Input: part model. Units: mm. Frame: model coordinates. A direction names the side the tool comes from. Coordinates: 2 decimals unless noted, no trailing zeros. Loops run counter-clockwise (first coordinate to the right, second up) from the corner with the lowest first, then second, coordinate; pieces in that order, holes last.
(1) Mould query, pull axis X, two halves, no side actions, for faces 1 (the face through (-18.516, -32.709, 1.61)), 2 (the face through (-38.944, 18.34, 1.61)), 3 (the face through (-0.72, -32.66, 1.61)). Classes: released by +X, released by -X, zero draft, split by the parting line, or undercut.
(2) Contact query for flat-ended pins moving along their axis: P1, Ø1.7, axis at x = -2.38, y = 19.05, coming from the +Z side; P2, Ø1.6, axis at x = -11, z = 1.5, coming from the +Y side; P3, Ø1, axis at y = 69.5, z = 1.5, coming from the -X side; P4, Ø1.5, axis at x = -13, z = 0.5, coming from the +Y side. Output: stop coordinate, or through.
(3) Line query: L1, parallel to Y at x = -24.5, z = 0.35; L2, parallel to Y at x = -29, z = 1.6; L3, parallel to X at y = 77.5, z = 1.8. Output: solid intervals per line, ascending.
(4) Section B-B, the plane y = 69.85. Return loops of the section in (x, z) (1 decimal), then the cut area to 3 significant figures.
(5) Section A-A, the plane y = -16. Return loops of the section in (x, z) (1 decimal), then the cut area to 3 significant figures.
(6) Section C-C, the plane z = 2.4. Give the number of separate pieces and of enclosed holes in the cut face, then the cut area to 3 significant figures.
(7) Set-up query: faces 4 (the face through (-10, -29.206, 2)), 5 (the face through (-21.964, 82.011, 1.565)). Return all of +Z, -Z, +X, -X, +Y, -Y with unobstructed straight access to the full face (end or side cutting, diameter ignored); none if empty.
Autodesk Inventor part; units mm, degrees
ref_plane "YZ Plane" through (0, 0, 0) normal (1, 0, 0) x (0, 1, 0)
ref_plane "XZ Plane" through (0, 0, 0) normal (0, 1, 0) x (-1, 0, 0)
ref_plane "XY Plane" through (0, 0, 0) normal (0, 0, 1) x (1, 0, 0)
sketch "Sketch1" plane through (0, 0, 0) normal (0, 0, 1) x (1, 0, 0)
  line L0 (0, 0) -> (0, 136.2362)
  line L1 (-14.9636, 12.2907) -> (-39.7615, 17.7883)
  line L2 (-39.7615, 17.7883) -> (-33.7485, 44.911)
  line L3 (-33.7485, 44.911) -> (-8.9506, 39.4135)
  line L4 (-8.9506, 39.4135) -> (-14.9636, 12.2907)
  line L5 (-39.7615, 17.7883) -> (-8.9506, 39.4135) construction
  line L6 (-33.7485, 44.911) -> (-14.9636, 12.2907) construction
  circle A0 centre (-57.15, 12.7) radius 3.3401
  circle A1 centre (-57.15, 12.7) radius 6.35
  line L7 (0, 0) -> (-57.847, 6.3884)
  line L8 (-62.7825, 15.6321) -> (0, 136.2362)
  line L9 (-21.3496, 42.1622) -> (-27.3626, 15.0395) construction
  line L10 (0, 104.775) -> (-14.6831, 108.0302)
  line L11 (-35.4518, 7.8896) -> (-23.0529, 5.1408)
  line L12 (-23.0529, 5.1408) -> (-24.4273, -1.0586) construction
  line L13 (-24.4273, -1.0586) -> (-36.8262, 1.6901) construction
  line L14 (-36.8262, 1.6901) -> (-35.4518, 7.8896) construction
  line L15 (-35.4518, 7.8896) -> (-40.7688, 4.5023)
  line L16 (-8.9506, 39.4135) -> (-33.7485, 44.911)
  line L17 (-56.4271, 15.9609) -> (-57.15, 12.7) construction
  line L18 (-57.15, 12.7) -> (-60.4109, 13.4229) construction
  line L19 (-29.2523, 6.5152) -> (-36.1243, -24.4822) construction
  line L20 (-56.356, 15.9443) -> (-9.0672, 106.7852)
  line L21 (-35.1857, 56.612) -> (0, 48.8115)
  line L22 (-4.7625, 49.8673) -> (-4.7625, 105.8308)
  line L23 (-30.3721, 55.5448) -> (-10.3247, 94.0556)
  line L24 (-10.3247, 94.0556) -> (-4.7625, 92.8225)
  circle A2 centre (-17.3978, 7.9523) radius 2
  line L25 (0, 13.4938) -> (-4.7625, 13.4937) construction
  line L26 (-4.7625, 13.4937) -> (-4.7625, 24.6063) construction
  line L27 (-4.7625, 24.6063) -> (0, 24.6063) construction
  line L28 (0, 24.6063) -> (0, 13.4938) construction
  line L29 (-4.7625, 19.05) -> (0, 19.05) construction
  circle A3 centre (-2.3812, 19.05) radius 1.4224
  line L30 (-4.7625, 57.15) -> (0, 57.15) construction
  circle A4 centre (-2.3813, 57.15) radius 1.4224
  circle A5 centre (-2.3813, 63.5) radius 1.4224
  circle A6 centre (-2.3813, 69.85) radius 1.4224
  circle A7 centre (-2.3813, 76.2) radius 1.4224
  line L31 (-22.792, 92.4532) -> (-17.8635, 89.8876)
  circle A8 centre (-57.15, 12.7) radius 9.525 construction
  line L32 (-14.7625, 0.7937) -> (-4.7625, 0.7938)
  line L33 (-4.7625, 0.7938) -> (-4.7625, -29.2062)
  line L34 (-4.7625, -29.2062) -> (-14.7625, -29.2062)
  line L35 (-14.7625, -29.2062) -> (-14.7625, 0.7937)
  line L36 (-14.7625, 0.7937) -> (-4.7625, -29.2062) construction
  line L37 (-4.7625, 0.7938) -> (-14.7625, -29.2062) construction
  line L38 (-19.05, -33.3375) -> (0, -33.3375)
  line L39 (0, -33.3375) -> (0, 0)
  line L40 (-23.0529, 5.1408) -> (-19.05, -33.3375)
  circle A9 centre (-17.3978, 7.9523) radius 6.5 construction
  line L41 (-22.7129, 14.0087) -> (-24.6027, 5.4844) construction
  line L42 (-17.3978, 7.9523) -> (-23.8273, 9.3776) construction
  line L43 (-33.8287, 59.2189) -> (-45.835, 5.0618)
  point P0 (-24.3561, 28.6009)
  point P1 (-23.6144, 2.6079)
  point P2 (-36.3119, 4.0101)
  point P3 (-54.945, 18.6549)
  point P4 (0, 48.8115)
  point P5 (-24.3561, 28.6009)
  point P6 (-9.7625, -14.2062)
  dimension "d14" = 27.7812
  dimension "d15" = 25.4
  dimension "d16" = 12.5
  dimension "d17" = 6.6802
  dimension "d19" = 57.15
  dimension "d22" = 12.7
  dimension "d26" = 102.5
  dimension "d29" = 6.35
  dimension "d31" = 6.35
  dimension "d35" = 28.575
  dimension "d38" = 31.75
  dimension "d55" = 4.7625
  dimension "d56" = 4.7625
  dimension "d60" = 12.7
  dimension "d66" = 4
  dimension "d72" = 8.7312
  dimension "d80" = 104.775
  dimension "d85" = 4.7625
  dimension "d86" = 11.1125
  dimension "d87" = 2.8448
  dimension "d88" = 19.05
  dimension "d89" = 2.8448
  dimension "d90" = 38.1
  dimension "d93" = 6.35
  dimension "d104" = 27.5
  dimension "d105" = 5.5563
  dimension "d106" = 19.05
  dimension "d111" = 19.05
  dimension "d112" = 10
  dimension "d113" = 30
  dimension "d114" = 4.7625
  dimension "d115" = 0.7937
  dimension "d117" = 19.05
  dimension "d119" = 11.1125
  dimension "d120" = 12.7
  dimension "d121" = 33.3375
  dimension "d122" = 45
  dimension "d123" = 13
  dimension "d124" = 4.7625
  dimension "d125" = 4.7625
  dimension "d126" = 3.175
extrude "Extrusion1" add sketch "Sketch1" along normal blind 3.175 contours L7 L33 L32 L40 L11 L15 L43 L21 L0 | L39 L38 L40 L7 L32 L35 L34 L33 | L21 L22 L10 L0 | L22 L24 L23 L21 L43 L20 L10
fillet "Fillet1" radius 2.3813 17 edges at (-39.7615, 17.7883, 1.5875) (-14.9636, 12.2907, 1.5875) (-23.0529, 5.1408, 1.5875) (-35.4518, 7.8896, 1.5875) (-40.7688, 4.5023, 1.5875) (-4.7625, 92.8225, 1.5875) (-30.3721, 55.5448, 1.5875) (-4.7625, 49.8673, 1.5875) (-33.7485, 44.911, 1.5875) (-8.9506, 39.4135, 1.5875) (-19.05, -33.3375, 1.5875) (0, -33.3375, 1.5875) (-10.3247, 94.0556, 1.5875) (-33.8287, 59.2189, 1.5875) (-45.835, 5.0618, 1.5875) (-9.0672, 106.7852, 1.5875) (0, 104.775, 1.5875)
fillet "Fillet6" radius 1 4 edges at (-4.7625, 0.7938, 1.5875) (-14.7625, 0.7937, 1.5875) (-14.7625, -29.2062, 1.5875) (-4.7625, -29.2062, 1.5875)
equation "\"d56\" = d55"
properties part number "Uprights" material "Stainless Steel"
Report:
1. face 1: released by -X
1. face 2: undercut
1. face 3: released by +X
2. P1: passes through
2. P2: stops at y = 104.61
2. P3: stops at x = -28.74
2. P4: stops at y = 100.67
3. L1: y = 5.45 to 14.4, 42.86 to 54.24, 66.83 to 77.14
3. L2: y = 6.46 to 15.4, 43.86 to 56.22, 58.17 to 68.49
3. L3: x = -24.31 to -18.94, -4.76 to -2.96, -1.8 to 0
4. outline: (-28.3, 0) - (-22.9, 0) - (-22.9, 3.2) - (-28.3, 3.2) - close; (-4.8, 0) - (-3.8, 0) - (-3.8, 3.2) - (-4.8, 3.2) - close; (-1, 0) - (0, 0) - (0, 3.2) - (-1, 3.2) - close
4. area: 23.1 mm2
5. outline: (-20.9, 0) - (-14.8, 0) - (-14.8, 3.2) - (-20.9, 3.2) - close; (-4.8, 0) - (0, 0) - (0, 3.2) - (-4.8, 3.2) - close
5. area: 34.5 mm2
6. separate pieces: 1
6. enclosed holes: 9
6. area: 2,240 mm2
7. face 4: +Z, -Z
7. face 5: +Z, -Z, -X, +Y
